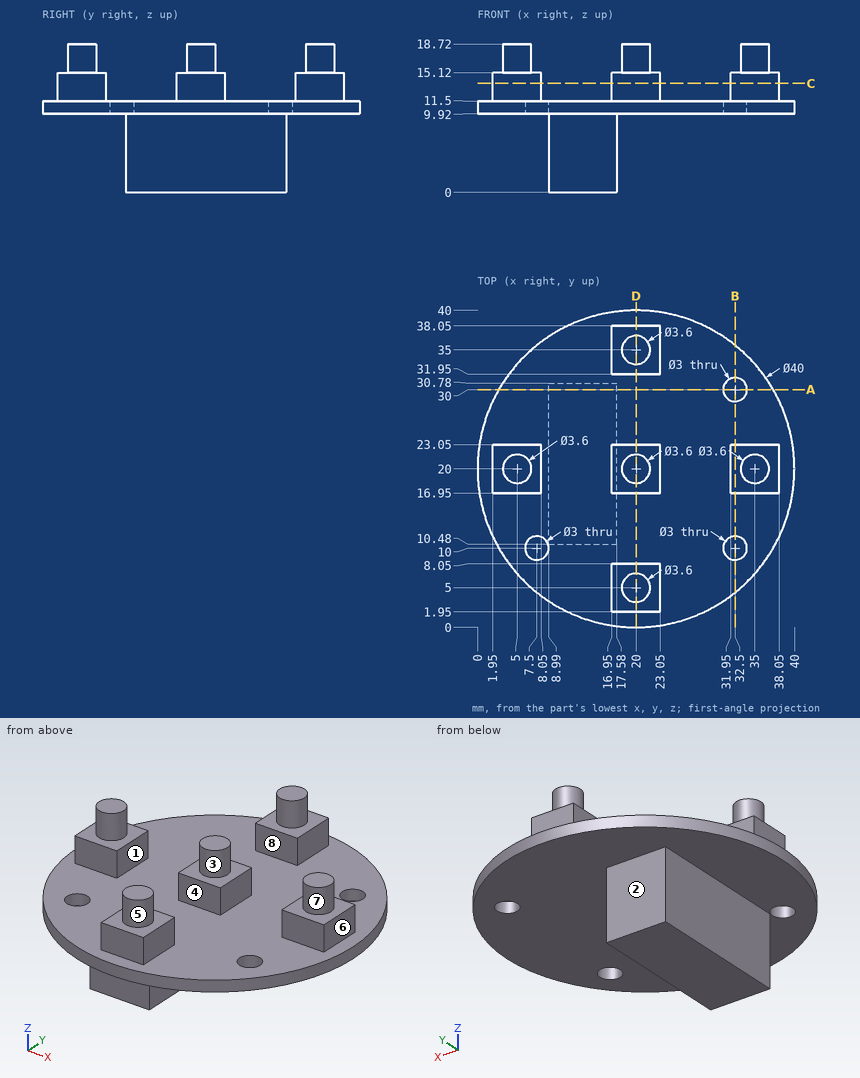
Can you work these out from the drawing? Everything is in mm from the part's minimum corner. A direction names the side the tool comes from. Round coordinates to 2 decimals unless told otherwise and drop trailing zeros. Loops run counter-clockwise (first coordinate to the right, second up) from the corner with the lowest first, then second, coordinate; pieces in that order, holes last. Notation, with made-up numbers: M 35,41 L 54,41 A28 ccw 54,69 Z; hole C 13,77 d4. An arc over 180 degrees is marked long. Write item = value, one per line.
1. I want a section at A-A, the plane y = 30. Write out the boundary of the cut face in (x, z).
Results below:
outline = M 2.68,9.92 L 8.99,9.92 L 8.99,0 L 17.58,0 L 17.58,9.92 L 31,9.92 L 31,11.5 L 2.68,11.5 Z; M 34,9.92 L 37.32,9.92 L 37.32,11.5 L 34,11.5 Z
2. Thinking about a two-plate mould opening in X: for the marked faces 5, 6, 7 and 8, which applies, +X half, -X half, draft (parallel to the pull), parting line (faces both ways), or undercut?
Results below:
face_5 = parting line
face_6 = +X half
face_7 = undercut
face_8 = draft
3. I want a section at C-C, the plane z = 13.75. Write out the boundary of the cut face in (x, y), and give its area (3 significant figures).
Results below:
outline = M 1.95,16.95 L 8.05,16.95 L 8.05,23.05 L 1.95,23.05 Z; M 16.95,1.95 L 23.05,1.95 L 23.05,8.05 L 16.95,8.05 Z; M 16.95,16.95 L 23.05,16.95 L 23.05,23.05 L 16.95,23.05 Z; M 16.95,31.95 L 23.05,31.95 L 23.05,38.05 L 16.95,38.05 Z; M 31.95,16.95 L 38.05,16.95 L 38.05,23.05 L 31.95,23.05 Z
area = 186 mm²
4. I want a section at D-D, the plane x = 20. Write out the boundary of the cut face in (y, z).
Results below:
outline = M 0,9.92 L 40,9.92 L 40,11.5 L 38.05,11.5 L 38.05,15.12 L 36.8,15.12 L 36.8,18.72 L 33.2,18.72 L 33.2,15.12 L 31.95,15.12 L 31.95,11.5 L 23.05,11.5 L 23.05,15.12 L 21.8,15.12 L 21.8,18.72 L 18.2,18.72 L 18.2,15.12 L 16.95,15.12 L 16.95,11.5 L 8.05,11.5 L 8.05,15.12 L 6.8,15.12 L 6.8,18.72 L 3.2,18.72 L 3.2,15.12 L 1.95,15.12 L 1.95,11.5 L 0,11.5 Z
5. I need wall thicknesses on probe 1 along X at (y, z) = (19, 16); probe 2 along Y at (x, z) = (32.5, 10.85); probe 3 along Z at (x, y) = (16, 11). Which ranges of each line are inside material? Lowest first, please.
Results below:
probe_1 = 3.5 to 6.5, 18.5 to 21.5, 33.5 to 36.5
probe_2 = 4.39 to 8.5, 11.5 to 28.5, 31.5 to 35.61
probe_3 = 0 to 11.5
6. Will these pins go through, and if not, where does the flat tip stop? P1, Ø3, axis at x = 19, z = 13.5, coming from the +Y side; P2, Ø1.1, axis at y = 21.5, z = 13, coming from the -X side; P3, Ø1.8, axis at x = 21, z = 13.5, coming from the -Y side.
Results below:
P1 = 38.05
P2 = 1.95
P3 = 1.95
7. Which directions (+Z, -Z, +X, -X, +Y, -Y) give clear straight access to the entire face, cutting with the end or side of a thin tool? Please do the marked faces 1, 2, 3 and 4.
Results below:
face_1 = +Z, +Y, -Y
face_2 = -Z, +X, -X, +Y
face_3 = +Z
face_4 = +Z, +X, -X
8. I want a section at B-B, the plane x = 32.5. Write out the boundary of the cut face in (y, z).
Results below:
outline = M 4.39,9.92 L 8.5,9.92 L 8.5,11.5 L 4.39,11.5 Z; M 11.5,9.92 L 28.5,9.92 L 28.5,11.5 L 23.05,11.5 L 23.05,15.12 L 16.95,15.12 L 16.95,11.5 L 11.5,11.5 Z; M 31.5,9.92 L 35.61,9.92 L 35.61,11.5 L 31.5,11.5 Z
